from build123d import *

# Parameters (mm, degrees)
F0_W     = 101.6
F0_H     = 711.2
F1_DEPTH = 101.6
F2_W     = 101.6
F2_H     = 50.8
F3_DEPTH = 50.8
F5_DEPTH = 101.6


with BuildPart() as f1:
    # F0 (on Front) → F1 (new body)
    with BuildSketch(Plane.XZ):
        Rectangle(F0_W, F0_H)
    extrude(amount=F1_DEPTH)

    # F2 (on face) → F3 (cut)
    with BuildSketch(Plane.XY.offset(355.6)):
        with Locations((0, -50.8)):
            Rectangle(F2_W, F2_H)
    extrude(amount=-F3_DEPTH, mode=Mode.SUBTRACT)

    # F4 (on face) → F5 (cut)
    with BuildSketch(Plane.XZ.offset(101.6)):
        Polygon((0, -101.6), (25.4, -101.6), (25.4, -50.8), (-25.4, -50.8), (-25.4, -101.6), align=None)
    extrude(amount=-F5_DEPTH, mode=Mode.SUBTRACT)


solid = f1.part
Could you check a few things on this model? Use its own coordinates, in mm. A direction names the side the tool comes from. Round coordinates to 2 decimals unless told otherwise and drop trailing zeros. Write each loop counter-clockwise with the first axis right and the second up, starting at its lowest first coordinate (ties: lowest second). Pieces come first, ordered by that corner, then holes. Notation, with made-up numbers: (21, 31.5) - (56, 31.5) arc R7 ccw to (56, 36.5) - close; hole circle Ø1 at (-6.75, 14.5). An arc over 180 degrees is marked (long way). Put each result on its own line as item: value. Start each with the question number.
(1) I want a section at A-A, the plane y = -32. Please give me the cut outline in (x, z), plus the area to 3 significant figures.
(2) I want a section at C-C, the plane x = 36. Please give me the cut outline in (y, z), plus the area to 3 significant figures.
(3) I need wall thicknesses on probe 1 along Z at (x, y) = (-6.5, -52.5); probe 2 along Z at (x, y) = (-24.5, -97); probe 3 along Z at (x, y) = (-31, -65). Which ranges of each line are inside material? Lowest first, please.
(4) Will this pin go through, and if not, where does the flat tip stop? pin 1 (4 mm diameter, centred on x = 26.5, y = -69, fed in from +Z).
(5) For faces 4 (the flat face through (-1, -25.4, 331)), 5 (the flat face through (-1, -50, -355.6)), 6 (the flat face through (0, -52, -50.8)), which set-ups out of +Z, -Z, +X, -X, +Y, -Y let a thin tool reach every point of the face, with its end or its side?
(6) I want a section at B-B, the plane x = -14.5. Please give me the cut outline in (y, z).
(7) I want a section at D-D, the plane y = -92. Please give me the cut outline in (x, z).
(8) Thinking about a two-plate mould opening in Z: for faces 1 (the flat face through (-1, -76.2, 331)), 2 (the flat face through (0, -52, -101.6)), 3 (the flat face through (-1, -50, 304.8)), which applies, released by +Z, released by -Z, zero draft, split by the parting line, or undercut?
Here are the results:
1. outline: (-50.8, -355.6) - (50.8, -355.6) - (50.8, 304.8) - (-50.8, 304.8) - close; hole (-25.4, -101.6) - (25.4, -101.6) - (25.4, -50.8) - (-25.4, -50.8) - close
1. area: 64,500 mm^2
2. outline: (-101.6, -355.6) - (0, -355.6) - (0, 355.6) - (-25.4, 355.6) - (-25.4, 304.8) - (-76.2, 304.8) - (-76.2, 355.6) - (-101.6, 355.6) - close
2. area: 69,700 mm^2
3. probe 1: z = -355.6 to -101.6, -50.8 to 304.8
3. probe 2: z = -355.6 to -101.6, -50.8 to 355.6
3. probe 3: z = -355.6 to 304.8
4. pin 1: stops at z = 304.8
5. face 4: +Z, +X, -X
5. face 5: -Z, +X, -X, +Y, -Y
5. face 6: +Y, -Y
6. outline: (-101.6, -355.6) - (0, -355.6) - (0, -101.6) - (-101.6, -101.6) - close; (-101.6, -50.8) - (0, -50.8) - (0, 355.6) - (-25.4, 355.6) - (-25.4, 304.8) - (-76.2, 304.8) - (-76.2, 355.6) - (-101.6, 355.6) - close
7. outline: (-50.8, -355.6) - (50.8, -355.6) - (50.8, 355.6) - (-50.8, 355.6) - close; hole (-25.4, -101.6) - (25.4, -101.6) - (25.4, -50.8) - (-25.4, -50.8) - close
8. face 1: zero draft
8. face 2: undercut
8. face 3: released by +Z
